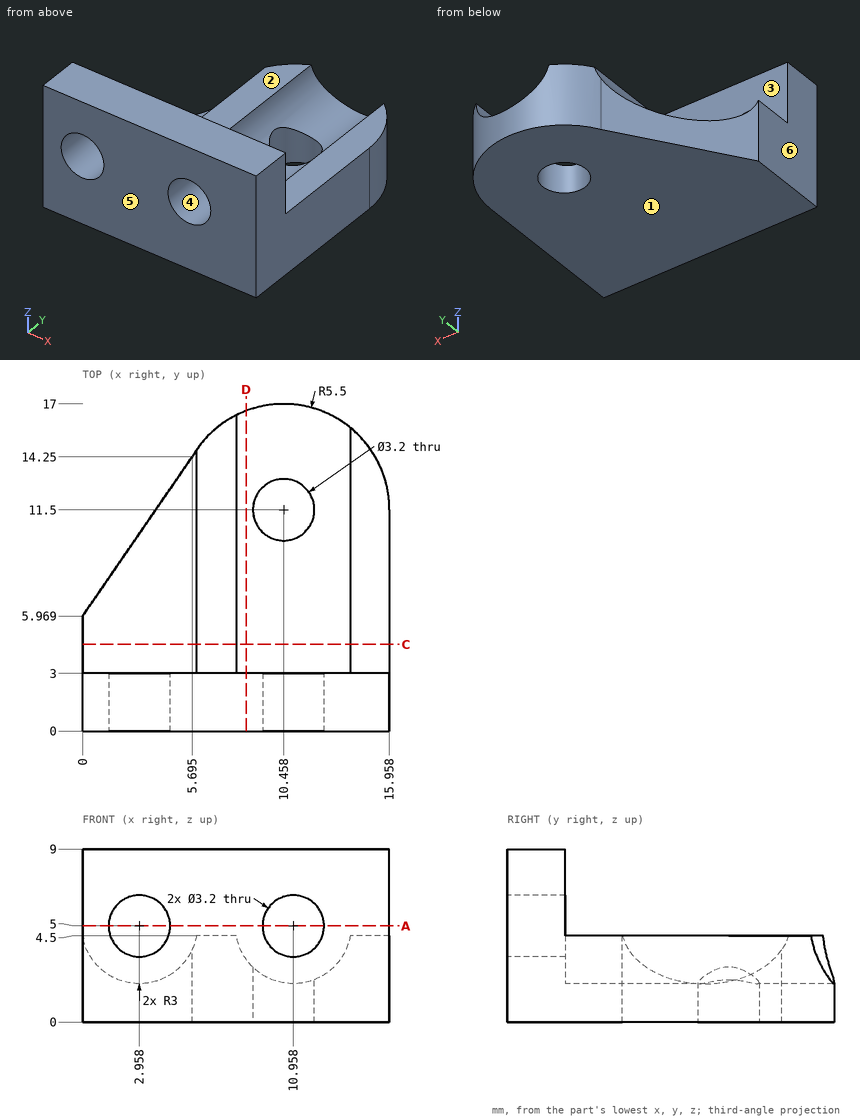
Geometry check sheet. Reference: drawing and pictorial views, mm from the part's lowest x, y, z. A direction names the side the tool comes from. Round coordinates to 2 decimals unless told otherwise and drop trailing zeros. Order: outer loops, then holes, each group sorted by start corner. A loop starts at its lowest first (then second) coordinate and runs counter-clockwise, first axis right, second up. Notation, with made-up numbers: M 21.25,79.5 L 57.25,79.5 A20 ccw 57.25,116.5 Z; hole C 12.25,-35 d11. An arc over 180 degrees is marked long. Write item = value, one per line.
Q1. Section check A-A (z = 5). Enter the section's corners in (x, y), plus the area to 3 significant figures.
Answer block:
outline = M 0,0 L 1.36,0 L 1.36,3 L 0,3 Z; M 4.56,0 L 9.36,0 L 9.36,3 L 4.56,3 Z; M 12.56,0 L 15.96,0 L 15.96,3 L 12.56,3 Z
area = 28.7 mm^2
Q2. Release check for a two-part mould opening along X. For the marked faces 4, 5 and 6 record: released by +X, released by -X, zero draft, split by the parting line, or undercut.
Answer block:
face_4 = undercut
face_5 = zero draft
face_6 = released by -X
Q3. Set-up check for the marked faces 1, 2 and 3: record each of +Z, -Z, +X, -X, +Y, -Y from which the full face is reachable in a straight line by a thin tool's end or side.
Answer block:
face_1 = -Z, +X, -X, +Y, -Y
face_2 = +Z, +X, -X, +Y
face_3 = +Z, +Y
Q4. Section check C-C (y = 4.5). Enter the section's corners in (x, z).
Answer block:
outline = M 0,0 L 15.96,0 L 15.96,4.5 L 13.92,4.5 A3 cw 8,4.5 L 5.92,4.5 A3 cw 0,4.5 Z
Q5. Section check D-D (x = 8.5). Enter the section's corners in (y, z).
Answer block:
outline = M 0,0 L 16.64,0 L 16.64,3.28 L 3,3.28 L 3,9 L 0,9 Z
Q6. Scan lines: line 1 (X direction, y = 1.25, z = 4); line 2 (X direction, y = 5.25, z = 2.25) (1 decimal); line 3 (Y direction, x = 6.25, z = 6.5). Record each from-to range of solid material in increasing order.
Answer block:
line_1 = 0 to 1.71, 4.21 to 9.71, 12.21 to 15.96
line_2 = 0 to 1.8, 4.2 to 9.8, 12.2 to 16
line_3 = 0 to 3
Q7. Depth check by flat-ended pin: pin 1 Ø3 at (y, z) = (3.5, 5.5) entering from -X; pin 2 Ø1 at (x, y) = (7, 12.5) entering from +Z; pin 3 Ø1.9 at (x, z) = (2.958, 5) entering from -Y; pin 4 Ø2 at (x, z) = (13.5, 2) entering from +Y. Enter the tip coordinate at first touch or a pass-through.
Answer block:
pin_1 = 0
pin_2 = 4.5
pin_3 = through
pin_4 = 16.61
